```python
from build123d import *

# Parameters (mm, degrees)
F0_R     = 12.5
F0_R_2   = 7.5
F1_DEPTH = 25


with BuildPart() as f1:
    # F0 (on Top) → F1 (new body)
    with BuildSketch(Plane.XY):
        with BuildLine():
            ThreePointArc((72.567013, 61.385173), (-4.822021, 96.767399), (-86.213806, 71.941162))
            ThreePointArc((-86.213806, 71.941162), (-84.691521, 32.104929), (-46.76355, 44.381405))
            ThreePointArc((-46.76355, 44.381405), (-43.543389, 49.706376), (-38.439264, 53.266243))
            ThreePointArc((-38.439264, 53.266243), (2.871879, 60.669961), (43.341674, 49.551455))
            ThreePointArc((43.341674, 49.551455), (47.018279, 46.786549), (49.684065, 43.037454))
            ThreePointArc((49.684065, 43.037454), (72.480393, 38.049741), (72.567013, 61.385173))
        make_face()
        with Locations((-70.374292, 52.599244)):
            Circle(F0_R, mode=Mode.SUBTRACT)
        with Locations((63.097075, 49.752448)):
            Circle(F0_R_2, mode=Mode.SUBTRACT)
    extrude(amount=F1_DEPTH)


solid = f1.part
```
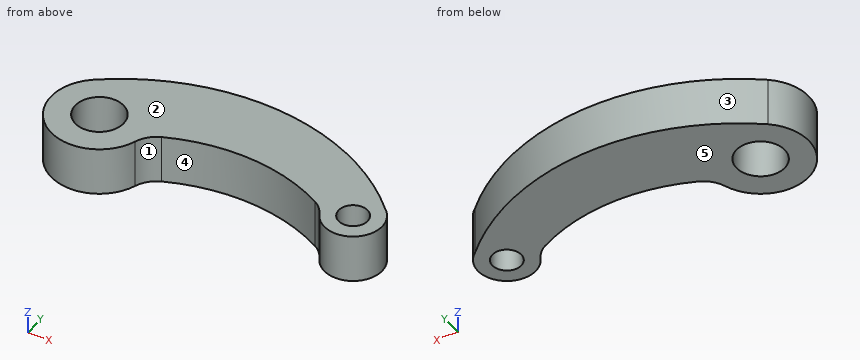
Geometry check sheet. Reference: the model listing, model coordinates, mm. Face numbers are marked on the shaded views. A direction names the side the tool comes from. Coordinates: 2 decimals unless noted, no trailing zeros. Loops run counter-clockwise (first coordinate to the right, second up) from the corner with the lowest first, then second, coordinate; pieces in that order, holes last.
Item 1: Go/stop test with flat-tipped pins: pin 1 Ø3 at (y, z) = (42.5, 7.5) entering from +X; pin 2 Ø1 at (y, z) = (39.5, 3) entering from +X; pin 3 Ø2 at (y, z) = (76, 4.5) entering from +X. Record where each tip stops, or that it passes through.
Item 2: Sectioned sample at C-C, the plane y = 69.5. Record the boundary of the cut face in (x, z).
Item 3: Access from +Z, -Z, +X, -X, +Y, -Y to the whole of each face (thin tool, end or side, straight path). Record for the marked faces 1 and 2.
Item 4: Sectioned sample at A-A, the plane x = -73. Record the boundary of the cut face in (y, z), then the cut area to 3 significant figures.
Item 5: Sectioned sample at D-D, the plane x = 11. Record the boundary of the cut face in (y, z), then the cut area to 3 significant figures.
Item 6: Sectioned sample at B-B, the plane z = 17. Record the boundary of the cut face in (x, y), then the cut area to 3 significant figures.
Item 7: Thickness scan on line 1 (X direction, y = 61, z = 1.75); line 2 (X direction, y = 47.5, z = 23); line 3 (Y direction, x = 62, z = 3.25). Record the ranges inside material, lowest first.
Item 8: Release check for a two-part mould opening along X. For the marked faces 3, 4 and 5 record: released by +X, released by -X, zero draft, split by the parting line, or undercut.
Check result:
1. pin 1: stops at x = 76.95
1. pin 2: stops at x = 74.49
1. pin 3: stops at x = 56.52
2. outline: (-88.8, 0) - (63.7, 0) - (63.7, 25) - (-88.8, 25) - close
3. face 1: +Z, -Z, -Y
3. face 2: +Z, +X, -X, +Y, -Y
4. outline: (27.74, 0) - (40.38, 0) - (40.38, 25) - (27.74, 25) - close; (64.82, 0) - (80.83, 0) - (80.83, 25) - (64.82, 25) - close
4. area: 716 mm2
5. outline: (59.95, 0) - (94.65, 0) - (94.65, 25) - (59.95, 25) - close
5. area: 868 mm2
6. outline: (-86.21, 71.94) arc R25 ccw (long way) to (-46.76, 44.38) arc R15 cw to (-38.44, 53.27) arc R95 cw to (43.34, 49.55) arc R15 cw to (49.68, 43.04) arc R15 ccw (long way) to (72.57, 61.39) arc R120 ccw to start; hole circle Ø25 at (-70.37, 52.6); hole circle Ø15 at (63.1, 49.75)
6. area: 6,050 mm2
7. line 1: x = -93.92 to -79.63, -61.12 to 73.02
7. line 2: x = -94.85 to -81.79, -58.96 to -45.25, 46.27 to 55.94, 70.25 to 77.93
7. line 3: y = 34.79 to 42.33, 57.17 to 70.88
8. face 3: split by the parting line
8. face 4: undercut
8. face 5: zero draft
